from build123d import *

# Parameters (mm, degrees)
F0_W     = 40
F0_H     = 112.7631144943
F1_DEPTH = 92.5
F2_W     = 167
F2_H     = 104
F3_DEPTH = 40
F4_W     = 19.1075097164
F4_H     = 21.1983466993
F5_DEPTH = 200
F7_DEPTH = 200


with BuildPart() as f1:
    # F0 (on Right) → F1 (new body, symmetric)
    with BuildSketch(Plane.YZ):
        Polygon((41.0424171991, 112.7631144943), (0, 0), (41.0424171991, 0), align=None)
        Polygon((41.0424171991, 0), (0, 0), (0, -15), (81.0424171991, -15), (81.0424171991, 0), align=None)
        with Locations((61.0424171991, 56.3815572472)):
            Rectangle(F0_W, F0_H)
    extrude(amount=F1_DEPTH, both=True)

    # F2 (on face) → F3 (cut)
    with BuildSketch(Plane(origin=(0, 0, 0), x_dir=(1, 0, 0), z_dir=(0, -0.9396926208, 0.3420201433))):
        with Locations((0, 60)):
            Rectangle(F2_W, F2_H)
    extrude(amount=-F3_DEPTH, mode=Mode.SUBTRACT)

    # F4 (on face) → F5 (cut)
    with BuildSketch(Plane.YZ.offset(92.5)):
        with Locations((90.5961720573, 102.1639411447)):
            Rectangle(F4_W, F4_H)
        Polygon((81.0424171991, 91.564767795), (81.0424171991, 112.7631144943), (41.0424171991, 112.7631144943), (33.3268499849, 91.564767795), align=None)
        Polygon((33.3268499849, 91.564767795), (41.0424171991, 112.7631144943), (33.0099269154, 112.7631144943), (33.0099269154, 91.564767795), align=None)
    extrude(amount=-F5_DEPTH, mode=Mode.SUBTRACT)

    # F6 (on face) → F7 (cut)
    with BuildSketch(Plane.YZ.offset(92.5)):
        Polygon((33.3268499849, 91.564767795), (7.8664632965, 21.6129302781), (31.3587788161, 13.0624266949), (59.9312942968, 91.564767795), align=None)
    extrude(amount=-F7_DEPTH, mode=Mode.SUBTRACT)


solid = f1.part
The model under review builds one solid part; all positions refer to its coordinate system, in mm. A direction names the side the tool comes from. Round coordinates to 2 decimals unless told otherwise and drop trailing zeros. Write each loop counter-clockwise with the first axis right and the second up, starting at its lowest first coordinate (ties: lowest second). Pieces come first, ordered by that corner, then holes. Notation, with made-up numbers: M 56.25,88.5 L 86.25,88.5 A16 cw 86.25,95.5 Z; hole C 31,53 d6. An arc over 180 degrees is marked long. Answer as CSV lines item,"result". Start each with the question number.
Q1. Consider section B-B, the plane y = 48. Give the boundary of the cut face in (x, z).
Q2. Consider section C-C, the plane z = 47. Give the boundary of the cut face in (x, y).
Q3. Tool access review of faces 4 (the face through (-92.5, 49, 27)), 5 (the face through (-87.937, 19.448, 17.398)), 6 (the face through (-83.5, 43, 35)): name each direction out of +Z, -Z, +X, -X, +Y, -Y from which nothing blocks a thin tool from reaching the whole face with its end or side.
Q4. Consider section A-A, the plane x = 30. Give the boundary of the cut face in (y, z).
Q5. Wall thickness on line 1 along X through (y, z) = (65, 74); line 2 along Z through (x, y) = (31, 17); line 3 along Z through (x, y) = (1, 5): over which ranges is each line inside the solid? List them lowest first.
Q6. The part is to be moulded in two halves that separate along Y. For faces 1 (the face through (-1.17, 21.27, 0.77)), 2 (the face through (21.85, 2.24, 6.15)), 3 (the face through (92.5, 49, 27)), say which applies: +Y half, -Y half, draft (parallel to the pull), parting line (faces both ways), or undercut.
Q7. Clearance check with flat-ended pins moving along their axes: P1, Ø1, axis at x = -55, z = 29, coming from the -Y side; P2, Ø6, axis at x = 44.5, z = 46.5, coming from the -Y side; P3, Ø2, axis at x = -9.5, y = 32.5, coming from the +Z side. State where each tip first meets the part, or that it passes through.
Result set:
1,outline,"M -92.5,-15 L 92.5,-15 L 92.5,58.78 L 83.5,58.78 L 83.5,14.93 L -83.5,14.93 L -83.5,58.78 L -92.5,58.78 Z"
2,outline,"M -92.5,43.71 L -83.5,43.71 L -83.5,59.67 L 83.5,59.67 L 83.5,43.71 L 92.5,43.71 L 92.5,81.04 L -92.5,81.04 Z"
3,face 4,"+Z, -Z, -X, +Y, -Y"
3,face 5,"+Z, +X, -X"
3,face 6,"+Z"
4,outline,"M 0,-15 L 81.04,-15 L 81.04,91.56 L 75.89,91.56 L 40.32,-6.16 L 2.74,7.52 L 0,0 Z"
5,line 1,"x = -92.5 to -83.5, 83.5 to 92.5"
5,line 2,"z = -15 to 2.33"
5,line 3,"z = -15 to 6.69"
6,face 1,"undercut"
6,face 2,"-Y half"
6,face 3,"draft"
7,P1,"stops at y = 52.94"
7,P2,"stops at y = 58.4"
7,P3,"stops at z = -2.95"
